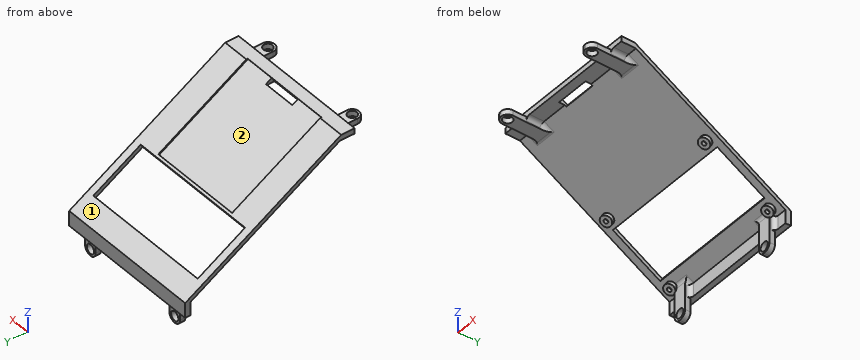
from build123d import *

# Parameters (mm, degrees)
BOSS_EXTRUDE1_DEPTH             = 55
CUT_EXTRUDE1_REACH              = 107.787
SKETCH3_W                       = 99
SKETCH3_H                       = 41
SKETCH4_W                       = 70
SKETCH4_H                       = 77
CUT_EXTRUDE2_DEPTH              = 1
SKETCH5_R                       = 4
SKETCH5_R_2                     = 1.5
BOSS_EXTRUDE2_DEPTH             = 3
SKETCH6_W                       = 10
SKETCH6_H                       = 4
BOSS_EXTRUDE3_DEPTH             = 15
BOSS_EXTRUDE3_DIRECTION_2_REACH = 124.058
CUT_EXTRUDE3_REACH              = 142.321
SKETCH7_R                       = 3.41
FILLET1_R                       = 3
FILLET2_R                       = 5
CUT_EXTRUDE4_REACH              = 112.137
SKETCH8_W                       = 25
SKETCH8_H                       = 5
SKETCH9_W                       = 10
SKETCH9_H                       = 4
BOSS_EXTRUDE4_DEPTH             = 15
BOSS_EXTRUDE4_DIRECTION_2_REACH = 149.117
CUT_EXTRUDE5_REACH              = 138.058
SKETCH10_R                      = 3.41
FILLET3_R                       = 3
FILLET4_R                       = 5


with BuildPart() as part:
    # Sketch2 → Boss-Extrude1 (new, symmetric)
    with BuildSketch(Plane(origin=(0, 0, 0), x_dir=(0, 0, -1), z_dir=(1, 0, 0))):
        Polygon((-52.121320344, -63.981493427), (16.76363182, 52.121320344), (27.878679656, 52.121320344), (27.878679656, 48.121320344), (17.878679656, 48.121320344), (-48.121320344, -63.119022696), (-48.121320344, -73.981493427), (-52.121320344, -73.981493427), align=None)
    extrude(amount=BOSS_EXTRUDE1_DEPTH, both=True)

    # Sketch3 → Cut-Extrude1 (cut, up to next)
    with BuildSketch(Plane(origin=(0, 6.214083509, 10.473587595), x_dir=(1, 0, 0), z_dir=(0, 0.5102589049122125, 0.8600208427461452)), mode=Mode.PRIVATE) as cut_extrude1_sk1:
        with Locations((0, 17.008093979)):
            Rectangle(SKETCH3_W, SKETCH3_H)
    cut_extrude1_tool1 = extrude(cut_extrude1_sk1.sketch, amount=-CUT_EXTRUDE1_REACH, mode=Mode.PRIVATE) & part.part
    add(cut_extrude1_tool1.solids().sort_by_distance((0, 20.841399, 1.795056))[0], mode=Mode.SUBTRACT)

    # Sketch4 → Cut-Extrude2 (cut)
    with BuildSketch(Plane(origin=(0, 6.214083509, 10.473587595), x_dir=(1, 0, 0), z_dir=(0, 0.5102589049122125, 0.8600208427461452))):
        with Locations((0, -43.991906021)):
            Rectangle(SKETCH4_W, SKETCH4_H)
    extrude(amount=-CUT_EXTRUDE2_DEPTH, mode=Mode.SUBTRACT)

    # Sketch5 → Boss-Extrude2 (add)
    # profile 1 of 4: a face of its own
    with BuildSketch(Plane(origin=(0, 4.683306794, 7.893525066), x_dir=(-1, 0, 0), z_dir=(0, -0.5102589049122127, -0.8600208427461451))):
        with Locations(Location((-46.5, 44.408093979, 0), (0, 0, 270))):
            Circle(SKETCH5_R)
        with Locations(Location((-46.5, 44.408093979, 0), (0, 0, 270))):
            Circle(SKETCH5_R_2, mode=Mode.SUBTRACT)
    # profile 2 of 4: a face of its own
    with BuildSketch(Plane(origin=(0, 4.683306794, 7.893525066), x_dir=(-1, 0, 0), z_dir=(0, -0.5102589049122127, -0.8600208427461451))):
        with Locations(Location((-46.5, -10.391906021, 0), (0, 0, 270))):
            Circle(SKETCH5_R)
        with Locations(Location((-46.5, -10.391906021, 0), (0, 0, 270))):
            Circle(SKETCH5_R_2, mode=Mode.SUBTRACT)
    # profile 3 of 4: a face of its own
    with BuildSketch(Plane(origin=(0, 4.683306794, 7.893525066), x_dir=(-1, 0, 0), z_dir=(0, -0.5102589049122127, -0.8600208427461451))):
        with Locations(Location((46.5, -10.391906021, 0), (0, 0, 270))):
            Circle(SKETCH5_R)
        with Locations(Location((46.5, -10.391906021, 0), (0, 0, 270))):
            Circle(SKETCH5_R_2, mode=Mode.SUBTRACT)
    # profile 4 of 4: a face of its own
    with BuildSketch(Plane(origin=(0, 4.683306794, 7.893525066), x_dir=(-1, 0, 0), z_dir=(0, -0.5102589049122127, -0.8600208427461451))):
        with Locations(Location((46.5, 44.408093979, 0), (0, 0, 270))):
            Circle(SKETCH5_R)
        with Locations(Location((46.5, 44.408093979, 0), (0, 0, 270))):
            Circle(SKETCH5_R_2, mode=Mode.SUBTRACT)
    extrude(amount=BOSS_EXTRUDE2_DEPTH)

    # Sketch6 → Boss-Extrude3 (add)
    with BuildSketch(Plane(origin=(0, 0, -27.878679656), x_dir=(-1, 0, 0), z_dir=(0, 0, -1))):
        with Locations((40, 46.121320344)):
            Rectangle(SKETCH6_W, SKETCH6_H)
        with Locations((-40, 46.121320344)):
            Rectangle(SKETCH6_W, SKETCH6_H)
    extrude(amount=BOSS_EXTRUDE3_DEPTH)

    # Sketch6 → Boss-Extrude3 direction 2 (add, up to next)
    with BuildSketch(Plane(origin=(0, 0, -27.878679656), x_dir=(-1, 0, 0), z_dir=(0, 0, -1)), mode=Mode.PRIVATE) as boss_extrude3_direction_2_sk1:
        with Locations((40, 46.121320344)):
            Rectangle(SKETCH6_W, SKETCH6_H)
    boss_extrude3_direction_2_tool1 = extrude(boss_extrude3_direction_2_sk1.sketch, amount=-BOSS_EXTRUDE3_DIRECTION_2_REACH, mode=Mode.PRIVATE) - part.part
    # Sketch6 → Boss-Extrude3 direction 2 (add, up to next)
    with BuildSketch(Plane(origin=(0, 0, -27.878679656), x_dir=(-1, 0, 0), z_dir=(0, 0, -1)), mode=Mode.PRIVATE) as boss_extrude3_direction_2_sk2:
        with Locations((-40, 46.121320344)):
            Rectangle(SKETCH6_W, SKETCH6_H)
    boss_extrude3_direction_2_tool2 = extrude(boss_extrude3_direction_2_sk2.sketch, amount=-BOSS_EXTRUDE3_DIRECTION_2_REACH, mode=Mode.PRIVATE) - part.part
    add(boss_extrude3_direction_2_tool1.solids().sort_by_distance((-40, 46.12132, -27.87868))[0])
    add(boss_extrude3_direction_2_tool2.solids().sort_by_distance((40, 46.12132, -27.87868))[0])

    # Sketch7 → Cut-Extrude3 (cut, up to next)
    with BuildSketch(Plane.XZ.offset(-44.121320344), mode=Mode.PRIVATE) as cut_extrude3_sk1:
        with Locations(Location((-40, -37.878679656, 0), (0, 0, 270))):
            Circle(SKETCH7_R)
    cut_extrude3_tool1 = extrude(cut_extrude3_sk1.sketch, amount=-CUT_EXTRUDE3_REACH, mode=Mode.PRIVATE) & part.part
    # Sketch7 → Cut-Extrude3 (cut, up to next)
    with BuildSketch(Plane.XZ.offset(-44.121320344), mode=Mode.PRIVATE) as cut_extrude3_sk2:
        with Locations(Location((40, -37.878679656, 0), (0, 0, 270))):
            Circle(SKETCH7_R)
    cut_extrude3_tool2 = extrude(cut_extrude3_sk2.sketch, amount=-CUT_EXTRUDE3_REACH, mode=Mode.PRIVATE) & part.part
    add(cut_extrude3_tool1.solids().sort_by_distance((-40, 44.12132, -37.87868))[0], mode=Mode.SUBTRACT)
    add(cut_extrude3_tool2.solids().sort_by_distance((40, 44.12132, -37.87868))[0], mode=Mode.SUBTRACT)

    # Fillet1
    fillet1_edges = [part.edges().sort_by_distance(p)[0] for p in [
        (-35, 46.121320344, -16.692059799),
        (35, 46.121320344, -16.692059799),
        (45, 48.121320344, -22.878679656),
        (35, 48.121320344, -22.878679656),
        (38.885828328, 44.121320344, -15.505439942),
        (-38.885828328, 44.121320344, -15.505439942),
        (-45, 48.121320344, -22.878679656),
        (-35, 48.121320344, -22.878679656),
    ]]
    fillet(fillet1_edges, radius=FILLET1_R)

    # Fillet2
    fillet2_edges = [part.edges().sort_by_distance(p)[0] for p in [
        (45, 46.121320344, -42.878679656),
        (35, 46.121320344, -42.878679656),
        (-35, 46.121320344, -42.878679656),
        (-45, 46.121320344, -42.878679656),
    ]]
    fillet(fillet2_edges, radius=FILLET2_R - 0.0001)  # a hair under: the kernel refuses the full size

    # Sketch8 → Cut-Extrude4 (cut, up to next)
    with BuildSketch(Plane(origin=(0, 5.703824604, 9.613566752), x_dir=(1, 0, 0), z_dir=(0, 0.5102589049122124, 0.8600208427461452)), mode=Mode.PRIVATE) as cut_extrude4_sk1:
        with Locations((0, -79.991906021)):
            Rectangle(SKETCH8_W, SKETCH8_H)
    cut_extrude4_tool1 = extrude(cut_extrude4_sk1.sketch, amount=-CUT_EXTRUDE4_REACH, mode=Mode.PRIVATE) & part.part
    add(cut_extrude4_tool1.solids().sort_by_distance((0, -63.090882, 50.430149))[0], mode=Mode.SUBTRACT)

    # Sketch9 → Boss-Extrude4 (add)
    with BuildSketch(Plane.XZ.offset(73.981493427)):
        with Locations((-40, 46.121320344)):
            Rectangle(SKETCH9_W, SKETCH9_H)
        with Locations((40, 46.121320344)):
            Rectangle(SKETCH9_W, SKETCH9_H)
    extrude(amount=BOSS_EXTRUDE4_DEPTH)

    # Boss-Extrude4 direction 2: up to this plane
    boss_extrude4_direction_2_end = Plane(origin=(55, 48.121320344, -17.878679656), z_dir=(0, 0.5102589049122126, 0.8600208427461451))
    # Sketch9 → Boss-Extrude4 direction 2 (add, up to the surface)
    with BuildSketch(Plane.XZ.offset(73.981493427), mode=Mode.PRIVATE) as boss_extrude4_direction_2_sk1:
        with Locations((-40, 46.121320344)):
            Rectangle(SKETCH9_W, SKETCH9_H)
    boss_extrude4_direction_2_tool1 = split(extrude(boss_extrude4_direction_2_sk1.sketch, amount=-BOSS_EXTRUDE4_DIRECTION_2_REACH, mode=Mode.PRIVATE), bisect_by=boss_extrude4_direction_2_end, keep=Keep.BOTH, mode=Mode.PRIVATE)
    add(boss_extrude4_direction_2_tool1.solids().sort_by_distance((-40, -73.981493, 46.12132))[0])
    # Sketch9 → Boss-Extrude4 direction 2 (add, up to the surface)
    with BuildSketch(Plane.XZ.offset(73.981493427), mode=Mode.PRIVATE) as boss_extrude4_direction_2_sk2:
        with Locations((40, 46.121320344)):
            Rectangle(SKETCH9_W, SKETCH9_H)
    boss_extrude4_direction_2_tool2 = split(extrude(boss_extrude4_direction_2_sk2.sketch, amount=-BOSS_EXTRUDE4_DIRECTION_2_REACH, mode=Mode.PRIVATE), bisect_by=boss_extrude4_direction_2_end, keep=Keep.BOTH, mode=Mode.PRIVATE)
    add(boss_extrude4_direction_2_tool2.solids().sort_by_distance((40, -73.981493, 46.12132))[0])

    # Sketch10 → Cut-Extrude5 (cut, up to next)
    with BuildSketch(Plane(origin=(0, 0, 44.121320344), x_dir=(-1, 0, 0), z_dir=(0, 0, -1)), mode=Mode.PRIVATE) as cut_extrude5_sk1:
        with Locations((40, -83.981493427)):
            Circle(SKETCH10_R)
    cut_extrude5_tool1 = extrude(cut_extrude5_sk1.sketch, amount=-CUT_EXTRUDE5_REACH, mode=Mode.PRIVATE) & part.part
    # Sketch10 → Cut-Extrude5 (cut, up to next)
    with BuildSketch(Plane(origin=(0, 0, 44.121320344), x_dir=(-1, 0, 0), z_dir=(0, 0, -1)), mode=Mode.PRIVATE) as cut_extrude5_sk2:
        with Locations(Location((-40, -83.981493427, 0), (0, 0, 180))):
            Circle(SKETCH10_R)
    cut_extrude5_tool2 = extrude(cut_extrude5_sk2.sketch, amount=-CUT_EXTRUDE5_REACH, mode=Mode.PRIVATE) & part.part
    add(cut_extrude5_tool1.solids().sort_by_distance((-40, -83.981493, 44.12132))[0], mode=Mode.SUBTRACT)
    add(cut_extrude5_tool2.solids().sort_by_distance((40, -83.981493, 44.12132))[0], mode=Mode.SUBTRACT)

    # Fillet3
    fillet3_edges = [part.edges().sort_by_distance(p)[0] for p in [
        (-45, -68.550258061, 48.121320344),
        (-35, -59.74810321, 46.121320344),
        (-35, -68.550258061, 48.121320344),
        (-40, -56.377183724, 44.121320344),
        (-45, -59.74810321, 46.121320344),
        (35, -68.550258061, 48.121320344),
        (45, -59.74810321, 46.121320344),
        (45, -68.550258061, 48.121320344),
        (40, -56.377183724, 44.121320344),
        (35, -59.74810321, 46.121320344),
    ]]
    fillet(fillet3_edges, radius=FILLET3_R)

    # Fillet4
    fillet4_edges = [part.edges().sort_by_distance(p)[0] for p in [
        (-45, -88.981493427, 46.121320344),
        (-35, -88.981493427, 46.121320344),
        (35, -88.981493427, 46.121320344),
        (45, -88.981493427, 46.121320344),
    ]]
    fillet(fillet4_edges, radius=FILLET4_R - 0.0001)  # a hair under: the kernel refuses the full size


solid = part.part
Could you check a few things on this model? Use its own coordinates, in mm. Face numbers are marked on the shaded views. Give positions to 0.01 mm unless a question says otherwise; leave off trailing zeros. Order: outer loops, then holes, each group sorted by start corner. A loop starts at its lowest first (then second) coordinate and runs counter-clockwise, first axis right, second up. Notation, with made-up numbers: (-14, 64) - (-9, 64) arc R12 ccw to (-9, 72) - close; hole circle Ø2 at (78.25, 70). An arc over 180 degrees is marked (long way). One line per item, written item: value. Start each with the question number.
1. Imagine slicing it at B-B on z = 20. List the corners of the cut face in (x, y) for me, plus the area to 3 significant figures.
2. Thinking about a two-plate mould opening in X: for the marked faces 1 and 2, which applies, +X half, -X half, draft (parallel to the pull), parting line (faces both ways), or undercut?
3. Imagine slicing it at A-A on x = -30. List the corners of the cut face in (y, z) for me.
4. For P1, Ø4.5, axis at y = -72, z = 45.5, coming from the -X side; P2, Ø10, axis at x = -22.5, y = -29.5, coming from the -Z side; P3, Ø8, axis at x = -40, y = -83.98, coming from the -Z side; P4, Ø4.5, axis at y = 46.5, z = -28.5, coming from the +X side, each with a flat end and sliding along its axis, tell me the tip position at first contact or that it passes through.
5. If I drill on probe 1 along Y at (x, z) = (-42.5, -23); probe 2 along Z at (x, y) = (-39.5, -29.5); probe 3 along Y at (x, z) = (29.5, -12.5), over which ranges is the centre line in solid material (lowest first)?
6. Imagine slicing it at C-C on y = -39. List the corners of the cut face in (x, z) for me.
Values:
1. outline: (-55, -15.72) - (55, -15.72) - (55, -9.84) - (35, -9.84) - (35, -11.8) - (-35, -11.8) - (-35, -9.84) - (-55, -9.84) - close
1. area: 510 mm²
2. face 1: draft
2. face 2: undercut
3. outline: (-73.98, 48.12) - (-63.12, 48.12) - (1.68, 9.68) - (3.21, 12.26) - (1.49, 13.28) - (0.98, 12.42) - (-65.24, 51.71) - (-64.99, 52.12) - (-73.98, 52.12) - close; (36.94, -11.25) - (48.12, -17.88) - (48.12, -27.88) - (52.12, -27.88) - (52.12, -16.76) - (38.47, -8.67) - close
4. P1: x = -46.55
4. P2: z = 25.21
4. P3: z = 44.12
4. P4: x = 55
5. probe 1: 44.12 to 52.12
5. probe 2: 28.17 to 31.66
5. probe 3: 39.06 to 44.94
6. outline: (-55, 33.81) - (55, 33.81) - (55, 37.3) - (35, 37.3) - (35, 36.14) - (-35, 36.14) - (-35, 37.3) - (-55, 37.3) - close
